Read the model definition and answer for the solid it produces. Units are mm, in the model's axes. Face numbers are marked on the shaded views. A direction names the side the tool comes from. Coordinates: 2 decimals unless noted, no trailing zeros. Write each loop counter-clockwise with the first axis right and the second up, starting at its lowest first coordinate (ties: lowest second). Pieces come first, ordered by that corner, then holes. Notation, with made-up numbers: (-15.5, 46.5) -> (-6.5, 46.5) arc R26 cw to (-6.5, 79.5) -> close; hole circle Ø11 at (28.25, 8.25). An arc over 180 degrees is marked (long way). Write item = value, one per line. Start each with the question number.
1) Find the intervals of material crossed by line 1 along X through (y, z) = (-89, 5); line 2 along Y through (x, z) = (53, 34.5); line 3 along Z through (x, y) = (61, -115), in increasing order. Write a range as from..to.
2) Section B-B (y = -65.5) is taken. Determine the outline of the cut face in (x, z).
3) A tool of negligible diameter and unlimited length cuts with its end or side. For the marked faces 1 and 2, from which of +Z, -Z, +X, -X, +Y, -Y can it reach the whole face along a straight path? Write none if from no direction.
4) Section A-A (z = 16.5) is taken. Determine the outline of the cut face in (x, y), plus the area to 3 significant figures.
5) Section C-C (x = 36) is taken. Determine the outline of the cut face in (y, z), plus the area to 3 significant figures.
6) Flat-ended cylindrical pins translate along their axes: pin 1 Ø1 at (x, y) = (101.5, -109) entering from +Z; pin 2 Ø1 at (x, y) = (64, -96) entering from +Z; pin 3 Ø0.6 at (y, z) = (-78.5, 36) entering from +X. Find the tip coordinate at first contact, or state that the pin passes through.
7) For a pull along X with two mould halves and no side action, classify the marked faces 3, 4, 5 and 6 as released by +X, released by -X, zero draft, split by the parting line, or undercut.
from build123d import *

# Parameters (mm, degrees)
F0_W      = 138
F0_H      = 125
F0_R      = 1.65
F1_DEPTH  = 3
F2_R      = 4
F3_DEPTH  = 1.5
F4_R      = 4
F5_DEPTH  = 3
F6_R      = 1.5
F7_DEPTH  = 6
F8_W      = 138
F8_H      = 125
F8_W_2    = 134
F8_H_2    = 121
F9_DEPTH  = 30
F11_DEPTH = 138
F13_DEPTH = 125


with BuildPart() as f1:
    # F0 (on Top) → F1 (new body)
    with BuildSketch(Plane.XY):
        with Locations((34.017931, -84.321183)):
            Rectangle(F0_W, F0_H)
        with Locations((-17.982069, -96.821183)):
            Circle(F0_R, mode=Mode.SUBTRACT)
        with Locations((86.017931, -96.821183)):
            Circle(F0_R, mode=Mode.SUBTRACT)
    extrude(amount=F1_DEPTH)

    # F2 (on face) → F3 (cut)
    with BuildSketch(Plane.XY.offset(3)):
        with Locations((-17.982069, -96.821183)):
            Circle(F2_R)
        with Locations((86.017931, -96.821183)):
            Circle(F2_R)
    extrude(amount=-F3_DEPTH, mode=Mode.SUBTRACT)

    # F4 (on face) → F5 (join)
    with BuildSketch(Plane.XY.offset(3)):
        with Locations((-21.482069, -127.321183)):
            Circle(F4_R)
        with Locations((-28.182069, -35.021183)):
            Circle(F4_R)
        with Locations((71.517931, -35.021183)):
            Circle(F4_R)
        with Locations((71.517931, -133.621183)):
            Circle(F4_R)
    extrude(amount=F5_DEPTH)

    # F6 (on face) → F7 (cut)
    with BuildSketch(Plane.XY.offset(6)):
        with Locations((-28.182069, -35.021183)):
            Circle(F6_R)
        with Locations((71.517931, -35.021183)):
            Circle(F6_R)
        with Locations((71.517931, -133.621183)):
            Circle(F6_R)
        with Locations((-21.482069, -127.321183)):
            Circle(F6_R)
    extrude(amount=-F7_DEPTH, mode=Mode.SUBTRACT)

    # F8 (on face) → F9 (join)
    with BuildSketch(Plane.XY.offset(3)):
        with Locations((34.017931, -84.321183)):
            Rectangle(F8_W, F8_H)
        with Locations((34.017931, -84.321183)):
            Rectangle(F8_W_2, F8_H_2, mode=Mode.SUBTRACT)
    extrude(amount=F9_DEPTH)

    # F10 (on face) → F11 (join)
    with BuildSketch(Plane.YZ.offset(103.017931)):
        Polygon((-146.821183, 40), (-146.821183, 33), (-144.821183, 33), (-144.821183, 34.5), (-145.821183, 35.5), (-145.821183, 37.5), (-144.821183, 38.5), (-144.821183, 40), align=None)
        Polygon((-23.821183, 40), (-23.821183, 38.5), (-22.821183, 37.5), (-22.821183, 35.5), (-23.821183, 34.5), (-23.821183, 33), (-21.821183, 33), (-21.821183, 40), align=None)
    extrude(amount=-F11_DEPTH)

    # F12 (on face) → F13 (join)
    with BuildSketch(Plane.XZ.offset(146.821183)):
        Polygon((-34.982069, 40), (-34.982069, 33), (-32.982069, 33), (-32.982069, 34.5), (-33.982069, 35.5), (-33.982069, 37.5), (-32.982069, 38.5), (-32.982069, 40), align=None)
    extrude(amount=-F13_DEPTH)


solid = f1.part
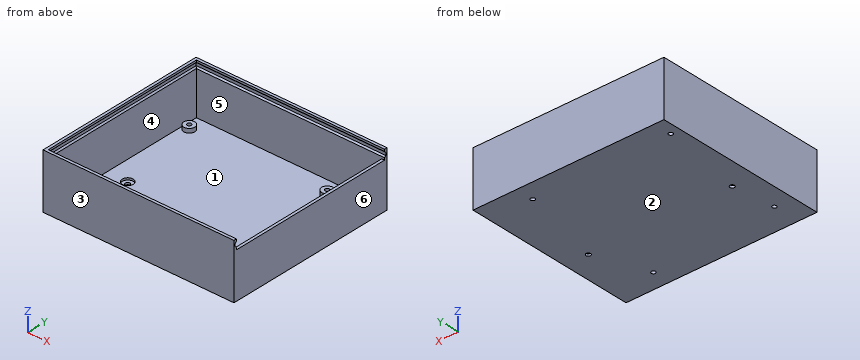
Answer key:
q1.line_1 = -34.98..-32.98, 101.02..103.02
q1.line_2 = -146.82..-144.82, -23.82..-21.82
q1.line_3 = 0..3
q2.outline = (-34.98, 0) -> (103.02, 0) -> (103.02, 33) -> (101.02, 33) -> (101.02, 3) -> (-32.98, 3) -> (-32.98, 34.5) -> (-33.98, 35.5) -> (-33.98, 37.5) -> (-32.98, 38.5) -> (-32.98, 40) -> (-34.98, 40) -> close
q3.face_1 = +Z
q3.face_2 = -Z, +X, -X, +Y, -Y
q4.outline = (-34.98, -146.82) -> (103.02, -146.82) -> (103.02, -21.82) -> (-34.98, -21.82) -> close; hole (-32.98, -144.82) -> (101.02, -144.82) -> (101.02, -23.82) -> (-32.98, -23.82) -> close
q4.area = 1,040 mm^2
q5.outline = (-146.82, 0) -> (-21.82, 0) -> (-21.82, 40) -> (-23.82, 40) -> (-23.82, 38.5) -> (-22.82, 37.5) -> (-22.82, 35.5) -> (-23.82, 34.5) -> (-23.82, 3) -> (-144.82, 3) -> (-144.82, 34.5) -> (-145.82, 35.5) -> (-145.82, 37.5) -> (-144.82, 38.5) -> (-144.82, 40) -> (-146.82, 40) -> close
q5.area = 517 mm^2
q6.pin_1 = 33
q6.pin_2 = 3
q6.pin_3 = -33.98
q7.face_3 = zero draft
q7.face_4 = undercut
q7.face_5 = undercut
q7.face_6 = released by +X
